Check sheet for the drawn part. Datum: minimum x, y, z corner. Units: mm. A direction names the side the tool comes from. Give positions to 0.01 mm unless a question says otherwise; leave off trailing zeros. Write each loop counter-clockwise with the first axis right and the second up, starting at its lowest first coordinate (ties: lowest second). Pieces come first, ordered by that corner, then holes. Notation, with made-up numbers: (32, 28.25) - (72, 28.25) arc R30 cw to (72, 52.25) - close; hole circle Ø6 at (28.5, 67). An arc over 180 degrees is marked (long way). Answer as a JSON object with one key per item and string values. Group by question number.
Item 1: Go/stop test with a flat-tipped pin: pin 1 (10 mm diameter, centred on x = 37.5, y = 18, fed in from -Z). Record where the tip stops, or that it passes through.
Item 2: Tool access check on the marked faces 1 and 2. Record the directions out of +Z, -Z, +X, -X, +Y, -Y that give a thin tool (end or side, any length) a straight path to the whole face; none if there is none.
Item 3: Sectioned sample at B-B, the plane z = 3.75. Record the boundary of the cut face in (x, y).
Item 4: Sectioned sample at A-A, the plane x = 5. Record the boundary of the cut face in (y, z).
Item 5: Scan lines: line 1 along Y through (x, z) = (40, 1.3); line 2 along X through (y, z) = (40, 3.5). Record each from-to range of solid material in increasing order. Write a range as [from, to].
Item 6: Draft check along Y on the marked faces 3, 4 and 5. Enter one of: +Y half, -Y half, draft (parallel to the pull), parting line (faces both ways), or undercut.
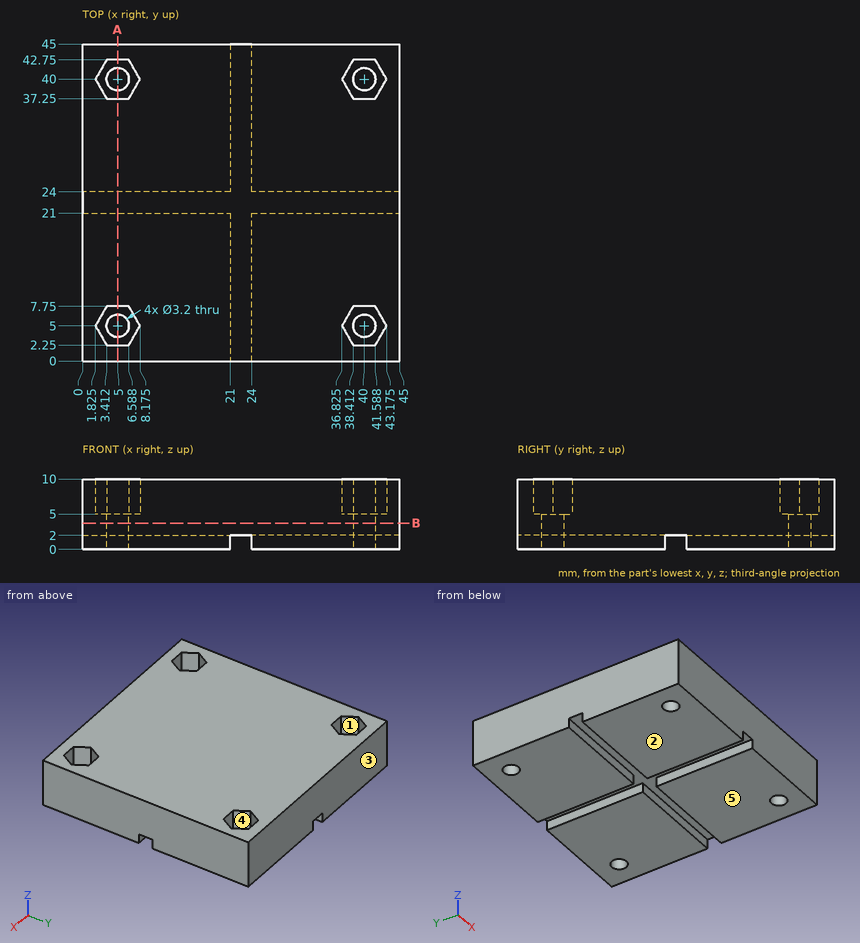
Geometry check:
{
 "1": {"pin 1": "z = 0"},
 "2": {"face 1": "+Z", "face 2": "-Z, +X, -X, +Y, -Y"},
 "3": {"outline": "(0, 0) - (45, 0) - (45, 45) - (0, 45) - close; hole circle Ø3.2 at (5, 5); hole circle Ø3.2 at (5, 40); hole circle Ø3.2 at (40, 5); hole circle Ø3.2 at (40, 40)"},
 "4": {"outline": "(0, 0) - (3.4, 0) - (3.4, 5) - (2.25, 5) - (2.25, 10) - (0, 10) - close; (6.6, 0) - (21, 0) - (21, 2) - (24, 2) - (24, 0) - (38.4, 0) - (38.4, 5) - (37.25, 5) - (37.25, 10) - (7.75, 10) - (7.75, 5) - (6.6, 5) - close; (41.6, 0) - (45, 0) - (45, 10) - (42.75, 10) - (42.75, 5) - (41.6, 5) - close"},
 "5": {"line 1": "[0, 3.4], [6.6, 21], [24, 38.4], [41.6, 45]", "line 2": "[0, 3.4], [6.6, 38.4], [41.6, 45]"},
 "6": {"face 3": "+Y half", "face 4": "undercut", "face 5": "draft"}
}
